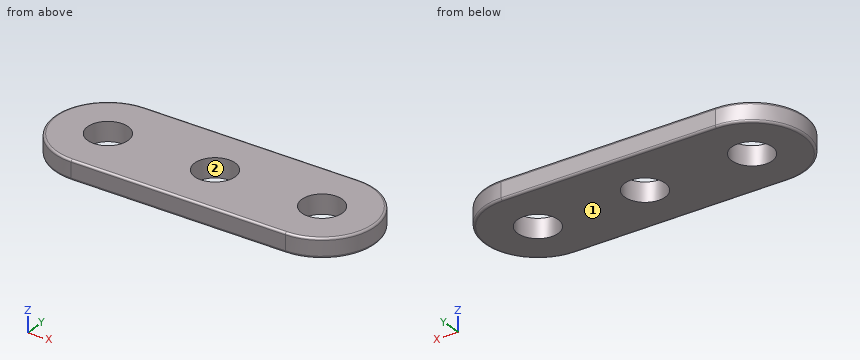
```python
from build123d import *

# Parameters (mm, degrees)
EXTRUDE1_DEPTH  = 2.286
SKETCH2_R       = 2.413
EXTRUDE2_DEPTH  = 21.21016566
LPATTERN1_COUNT = 3
LPATTERN1_PITCH = 12.7
FILLET1_R       = 0.254


with BuildPart() as part:
    # Sketch1 → Extrude1 (new body)
    with BuildSketch(Plane.XY):
        with BuildLine():
            Line((-12.7, 6.35), (12.7, 6.35))
            ThreePointArc((12.7, 6.35), (19.05, 0), (12.7, -6.35))
            Line((12.7, -6.35), (-12.7, -6.35))
            ThreePointArc((-12.7, -6.35), (-19.05, 0), (-12.7, 6.35))
        make_face()
    extrude(amount=EXTRUDE1_DEPTH)

    # Sketch2 → Extrude2 (cut, through all)
    with BuildSketch(Plane.XY.offset(2.286)):
        with Locations((-12.7, 0)):
            Circle(SKETCH2_R)
    extrude2 = extrude(amount=-EXTRUDE2_DEPTH, mode=Mode.SUBTRACT)

    # LPattern1: Extrude2 ×3
    with Locations(*[(i * LPATTERN1_PITCH, 0, 0) for i in range(1, LPATTERN1_COUNT)]):
        add(extrude2, mode=Mode.SUBTRACT)

    # Fillet1
    fillet1_edges = [part.edges().sort_by_distance(p)[0] for p in [
        (19.05, 0, 2.286),
        (0, 6.35, 2.286),
        (-19.05, 0, 2.286),
        (0, 6.35, 0),
        (19.05, 0, 0),
        (0, -6.35, 0),
        (-19.05, 0, 0),
        (0, -6.35, 2.286),
    ]]
    fillet(fillet1_edges, radius=FILLET1_R)


solid = part.part
```
Source: CAD feature listing. Evaluate the final solid. Frame: model axes, mm. Face numbers are marked on the shaded views. Coordinates: 2 decimals unless noted, no trailing zeros. Write each loop counter-clockwise with the first axis right and the second up, starting at its lowest first coordinate (ties: lowest second). Pieces come first, ordered by that corner, then holes. Notation, with made-up numbers: M 85.25,0 L 104.25,0 A28 cw 104.25,33 Z; hole C -37,52.5 d1. An arc over 180 degrees is marked long. Answer as a JSON object with one key per item and string values.
1. Cut plane B-B on y = 0. Output: boundary loops of the cut face in (x, z).
Evaluation:
{"outline": "M -19.05,0.25 A0.25 ccw -18.8,0 L -15.11,0 L -15.11,2.29 L -18.8,2.29 A0.25 ccw -19.05,2.03 Z; M -10.29,0 L -2.41,0 L -2.41,2.29 L -10.29,2.29 Z; M 2.41,0 L 10.29,0 L 10.29,2.29 L 2.41,2.29 Z; M 15.11,0 L 18.8,0 A0.25 ccw 19.05,0.25 L 19.05,2.03 A0.25 ccw 18.8,2.29 L 15.11,2.29 Z"}
2. Contact query for flat-ended pins moving along their axis: P1, Ø5.5, axis at x = -12.7, y = 0, coming from the +Z side; P2, Ø1, axis at x = 13.5, z = 1, coming from the -Y side. Output: stop coordinate, or through.
Evaluation:
{"P1": "z = 2.29", "P2": "y = -6.34"}
3. Cut plane D-D on x = 11. Output: boundary loops of the cut face in (y, z).
Evaluation:
{"outline": "M -6.35,0.25 A0.25 ccw -6.1,0 L -1.71,0 L -1.71,2.29 L -6.1,2.29 A0.25 ccw -6.35,2.03 Z; M 1.71,0 L 6.1,0 A0.25 ccw 6.35,0.25 L 6.35,2.03 A0.25 ccw 6.1,2.29 L 1.71,2.29 Z"}
4. Cut plane A-A on x = 0. Output: boundary loops of the cut face in (y, z), plus the area to 3 significant figures.
Evaluation:
{"outline": "M -6.35,0.25 A0.25 ccw -6.1,0 L -2.41,0 L -2.41,2.29 L -6.1,2.29 A0.25 ccw -6.35,2.03 Z; M 2.41,0 L 6.1,0 A0.25 ccw 6.35,0.25 L 6.35,2.03 A0.25 ccw 6.1,2.29 L 2.41,2.29 Z", "area": "17.9 mm^2"}
5. Ray query, L1, parallel to Y at x = 0, z = 1; L2, parallel to X at y = -0.75, z = 1.9. Return the intervals inside material, ascending.
Evaluation:
{"L1": "-6.35 to -2.41, 2.41 to 6.35", "L2": "-19.01 to -14.99, -10.41 to -2.29, 2.29 to 10.41, 14.99 to 19.01"}
6. Draft query along Y for the marked faces 1 and 2. Return one class per face: released by +Y, released by -Y, zero draft, split by the parting line, or undercut.
Evaluation:
{"face 1": "zero draft", "face 2": "undercut"}
7. Cut plane C-C on z = 1.65. Output: boundary loops of the cut face in (x, y).
Evaluation:
{"outline": "M -12.7,-6.35 L 12.7,-6.35 A6.35 ccw 12.7,6.35 L -12.7,6.35 A6.35 ccw Z; hole C -12.7,0 d4.83; hole C 0,0 d4.83; hole C 12.7,0 d4.83"}
